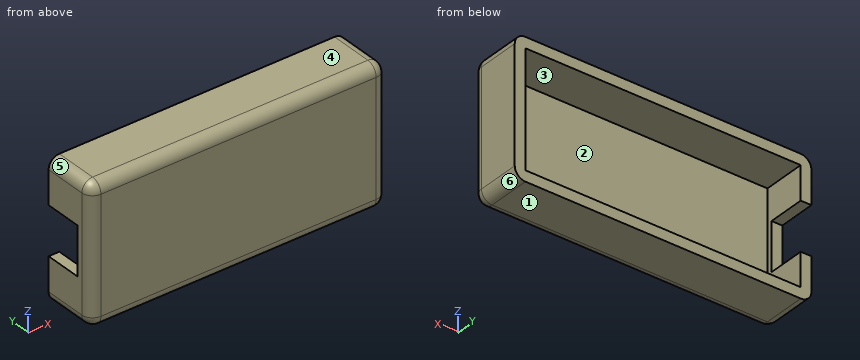
Autodesk Inventor part; units mm, degrees
ref_plane "YZ Plane" through (0, 0, 0) normal (1, 0, 0) x (0, 1, 0)
ref_plane "XZ Plane" through (0, 0, 0) normal (0, 1, 0) x (-1, 0, 0)
ref_plane "XY Plane" through (0, 0, 0) normal (0, 0, 1) x (1, 0, 0)
sketch "Sketch1" plane through (0, 0, 0) normal (0, 1, 0) x (-1, 0, 0)
  line L0 (0, 0) -> (51.5, 0)
  line L1 (51.5, 0) -> (51.5, -21.5)
  line L2 (51.5, -21.5) -> (0, -21.5)
  line L3 (0, -21.5) -> (0, 0)
  line L4 (53.5, 2) -> (-2, 2)
  line L5 (-2, 2) -> (-2, -23.5)
  line L6 (-2, -23.5) -> (53.5, -23.5)
  line L7 (53.5, -23.5) -> (53.5, 2)
  point P0 (49.5, -10.75)
  dimension "d0" = 51.5
  dimension "d1" = 21.5
  dimension "d2" = 2
  dimension "d3" = 2
  dimension "d4" = 2
  dimension "d5" = 2
extrude "Extrusion2" add sketch "Sketch1" against normal blind 2 contours L0 L1 L2 L3 | L7 L6 L5 L4
extrude "Extrusion3" add sketch "Sketch1" along normal blind 8
sketch "Sketch2" plane through (0, 8, 0) normal (0, 1, 0) x (1, 0, 0)
  line L0 (-51.5, 6.25) -> (-51.5, 15.25) construction
  line L1 (-51.5, 0) -> (-51.5, 21.5)
  line L2 (-51.5, 6.25) -> (-53.5, 6.25)
  line L3 (-53.5, -2) -> (-53.5, 23.5)
  line L4 (-51.5, 15.25) -> (-53.5, 15.25)
  point P0 (0, 0)
  point P1 (-51.5, 10.75)
  dimension "d20" = 9
extrude "Extrusion4" cut sketch "Sketch2" against normal blind 7
fillet "Fillet1" radius 2 8 edges at (2, 3, 2) (2, 3, -23.5) (-53.5, 3, 2) (-53.5, 3, -23.5) (-53.5, -2, -10.75) (-25.75, -2, -23.5) (2, -2, -10.75) (-25.75, -2, 2)
equation "\"d2\" = d4"
equation "\"d3\" = d4"
equation "\"d5\" = d4"
properties part number "case pico"
CAD build for the part. Positions are in the model's coordinates, mm. Face numbers are marked on the shaded views. A direction names the side the tool comes from. Give positions to 0.01 mm unless a question says otherwise; leave off trailing zeros. Order: outer loops, then holes, each group sorted by start corner. A loop starts at its lowest first (then second) coordinate and runs counter-clockwise, first axis right, second up. Notation, with made-up numbers: (-35, 24.25) -> (8, 24.25) arc R20 ccw to (8, 41.25) -> close; hole circle Ø4 at (79, 48). An arc over 180 degrees is marked (long way). Return JSON: item names as keys, results as strings.
Q1. Mould opens along X. For the marked faces 3, 4, 5 and 6 say: pulls with the +X half, pulls with the -X half, needs draft (parallel to the pull), parting line crosses it, or undercut.
Working result:
{"face 3": "undercut", "face 4": "needs draft", "face 5": "pulls with the -X half", "face 6": "pulls with the +X half"}
Q2. Saw through at A-A (z = -16.25). Write the cut outline in (x, y).
Working result:
{"outline": "(-53.5, 0) arc R2 ccw to (-51.5, -2) -> (0, -2) arc R2 ccw to (2, 0) -> (2, 8) -> (0, 8) -> (0, 0) -> (-51.5, 0) -> (-51.5, 8) -> (-53.5, 8) -> close"}
Q3. Flat gauge pins, fed straight in: pin 1 (1 mm diameter, centred on x = -52.5, z = -8.5, fed in from +Y); pin 2 (1.5 mm diameter, centred on x = -44.5, z = -16.5, fed in from +Y); pin 3 (1.6 mm diameter, centred on x = -52.5, y = 3.5, fed in from +Z). Where does each tip first touch, or does it go through?
Working result:
{"pin 1": "y = 1", "pin 2": "y = 0", "pin 3": "z = 1.99"}
Q4. Saw through at B-B (y = 5.5). Write the cut outline in (x, z).
Working result:
{"outline": "(-53.5, -21.5) arc R2 ccw to (-51.5, -23.5) -> (0, -23.5) arc R2 ccw to (2, -21.5) -> (2, 0) arc R2 ccw to (0, 2) -> (-51.5, 2) arc R2 ccw to (-53.5, 0) -> (-53.5, -6.25) -> (-51.5, -6.25) -> (-51.5, 0) -> (0, 0) -> (0, -21.5) -> (-51.5, -21.5) -> (-51.5, -15.25) -> (-53.5, -15.25) -> close"}
Q5. Drill centre lines: line 1 (Z direction, x = -5, y = 3.25); line 2 (X direction, y = 5.25, z = -2); line 3 (Y direction, x = -20.5, z = -8.75). Where is each one in solid material? Low to high.
Working result:
{"line 1": "-23.5 to -21.5, 0 to 2", "line 2": "-53.5 to -51.5, 0 to 2", "line 3": "-2 to 0"}
Q6. Saw through at C-C (x = -45). Write the cut outline in (y, z), then the cut area to 3 significant figures.
Working result:
{"outline": "(-2, -21.5) arc R2 ccw to (0, -23.5) -> (8, -23.5) -> (8, -21.5) -> (0, -21.5) -> (0, 0) -> (8, 0) -> (8, 2) -> (0, 2) arc R2 ccw to (-2, 0) -> close", "area": "81.3 mm²"}
Q7. Which spindle directions (+Z, -Z, +X, -X, +Y, -Y) get a long thin tool onto all of the face, cutting with end or side? Do the marked faces 1 and 2. Say none if no direction does.
Working result:
{"face 1": "-Z, +X, -X, +Y, -Y", "face 2": "+Y"}
